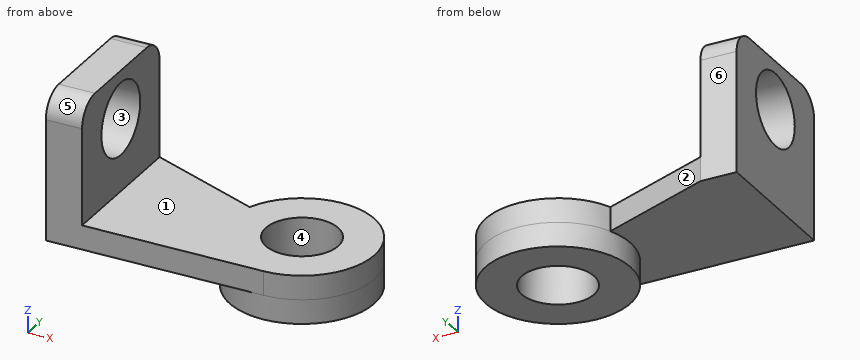
```python
from build123d import *

# Parameters (mm, degrees)
F0_R     = 38.1
F1_DEPTH = 25.4
F2_R     = 38.1
F3_DEPTH = 25.4
F4_R     = 38.1
F5_DEPTH = 38.1


with BuildPart() as f1:
    # F0 (on Top) → F1 (new body)
    with BuildSketch(Plane.XY):
        with BuildLine():
            ThreePointArc((0, -76.2), (53.8815367264, -53.8815367264), (76.2, 0))
            ThreePointArc((76.2, 0), (14.7223801552, 74.7642395973), (-70.5110635844, 28.8899621357))
            ThreePointArc((-70.5110635844, 28.8899621357), (-63.2765956525, -42.4560059665), (0, -76.2))
        make_face()
        Circle(F0_R, mode=Mode.SUBTRACT)
        with BuildLine():
            ThreePointArc((0, -76.2), (-63.2765956525, -42.4560059665), (-70.5110635844, 28.8899621357))
            Line((-70.5110635844, 28.8899621357), (-190.5, 76.2))
            Line((-190.5, 76.2), (-190.5, -76.2))
            Line((-190.5, -76.2), (0, -76.2))
        make_face()
    extrude(amount=F1_DEPTH)

    # F2 (on face) → F3 (join)
    with BuildSketch(Plane(origin=(0, 0, 0), x_dir=(1, 0, 0), z_dir=(0, 0, -1))):
        with BuildLine():
            ThreePointArc((-70.5110635844, -28.8899621357), (14.7223801552, -74.7642395973), (76.2, 0))
            ThreePointArc((76.2, 0), (53.8815367264, 53.8815367264), (0, 76.2))
            ThreePointArc((0, 76.2), (-63.2765956525, 42.4560059665), (-70.5110635844, -28.8899621357))
        make_face()
        Circle(F2_R, mode=Mode.SUBTRACT)
    extrude(amount=F3_DEPTH)

    # F4 (on face) → F5 (join)
    with BuildSketch(Plane(origin=(-190.5, 0, 0), x_dir=(0, -1, 0), z_dir=(-1, 0, 0))):
        with BuildLine():
            Line((-76.2, 0), (76.2, 0))
            Line((76.2, 0), (76.2, 127))
            ThreePointArc((76.2, 127), (68.7605122421, 144.9605122421), (50.8, 152.4))
            Line((50.8, 152.4), (-50.8, 152.4))
            ThreePointArc((-50.8, 152.4), (-68.7605122421, 144.9605122421), (-76.2, 127))
            Line((-76.2, 127), (-76.2, 0))
        make_face()
        with Locations((0, 101.6)):
            Circle(F4_R, mode=Mode.SUBTRACT)
        with BuildLine():
            Line((-76.2, 25.4), (76.2, 25.4))
            Line((76.2, 25.4), (76.2, 127))
            ThreePointArc((76.2, 127), (68.7605122421, 144.9605122421), (50.8, 152.4))
            Line((50.8, 152.4), (-50.8, 152.4))
            ThreePointArc((-50.8, 152.4), (-68.7605122421, 144.9605122421), (-76.2, 127))
            Line((-76.2, 127), (-76.2, 25.4))
        make_face()
        with Locations((0, 101.6)):
            Circle(F4_R, mode=Mode.SUBTRACT)
    extrude(amount=F5_DEPTH)


solid = f1.part
```
Work out the finished part from the listing and answer in its coordinate system (mm). Face numbers are marked on the shaded views. A direction names the side the tool comes from. Give positions to 0.01 mm unless a question says otherwise; leave off trailing zeros. Order: outer loops, then holes, each group sorted by start corner. A loop starts at its lowest first (then second) coordinate and runs counter-clockwise, first axis right, second up.
1. Each of these flat-tipped pins is pushed along its axis until it touches: P1, Ø10, axis at y = 38.5, z = 14.5, coming from the +X side; P2, Ø4, axis at x = -123, y = -1, coming from the -Z side; P3, Ø1, axis at y = -57.5, z = 83, coming from the +X side. Where does it stop, or does it pass through?
Result sheet:
P1: stops at x = 68.44
P2: stops at z = 0
P3: stops at x = -190.5
2. Section A-A, the plane y = 0 is taken. Determine the outline of the cut face in (x, z).
Result sheet:
outline: (-228.6, 0) - (-76.2, 0) - (-76.2, -25.4) - (-38.1, -25.4) - (-38.1, 25.4) - (-190.5, 25.4) - (-190.5, 63.5) - (-228.6, 63.5) - close; (-228.6, 139.7) - (-190.5, 139.7) - (-190.5, 152.4) - (-228.6, 152.4) - close; (38.1, -25.4) - (76.2, -25.4) - (76.2, 25.4) - (38.1, 25.4) - close
3. For the marked faces 1, 2 and 3, determine the directions among +Z, -Z, +X, -X, +Y, -Y from which every point of the face is accessible in a straight line to the end or side of a thin tool.
Result sheet:
face 1: +Z, +X, +Y, -Y
face 2: +Z, -Z, +Y
face 3: +X, -X
4. Section D-D, the plane y = -60 is taken. Determine the outline of the cut face in (x, z), and give its area (3 significant figures).
Result sheet:
outline: (-228.6, 0) - (-46.97, 0) - (-46.97, -25.4) - (46.97, -25.4) - (46.97, 25.4) - (-190.5, 25.4) - (-190.5, 150.68) - (-228.6, 150.68) - close
area: 14,200 mm2
5. Straight lines are drawn through the part: L1, parallel to Z at x = -198, y = 0; L2, parallel to X at y = 0, z = -5. For each, find the intervals that lie inside material, in ascending order.
Result sheet:
L1: z = 0 to 63.5, 139.7 to 152.4
L2: x = -76.2 to -38.1, 38.1 to 76.2
6. The mould has two halves that part along Y. Classify the marked faces 4, 5 and 6: released by +Y, released by -Y, zero draft, split by the parting line, or undercut.
Result sheet:
face 4: undercut
face 5: released by -Y
face 6: released by +Y
7. Section B-B, the plane z = 101.6 is taken. Determine the outline of the cut face in (x, y).
Result sheet:
outline: (-228.6, -76.2) - (-190.5, -76.2) - (-190.5, -38.1) - (-228.6, -38.1) - close; (-228.6, 38.1) - (-190.5, 38.1) - (-190.5, 76.2) - (-228.6, 76.2) - close
8. Section C-C, the plane x = -4.5 is taken. Determine the outline of the cut face in (y, z), and give its area (3 significant figures).
Result sheet:
outline: (-76.2, 0) - (-76.07, 0) - (-76.07, -25.4) - (-37.83, -25.4) - (-37.83, 25.4) - (-76.2, 25.4) - close; (37.83, -25.4) - (76.07, -25.4) - (76.07, 25.4) - (37.83, 25.4) - close
area: 3,890 mm2
